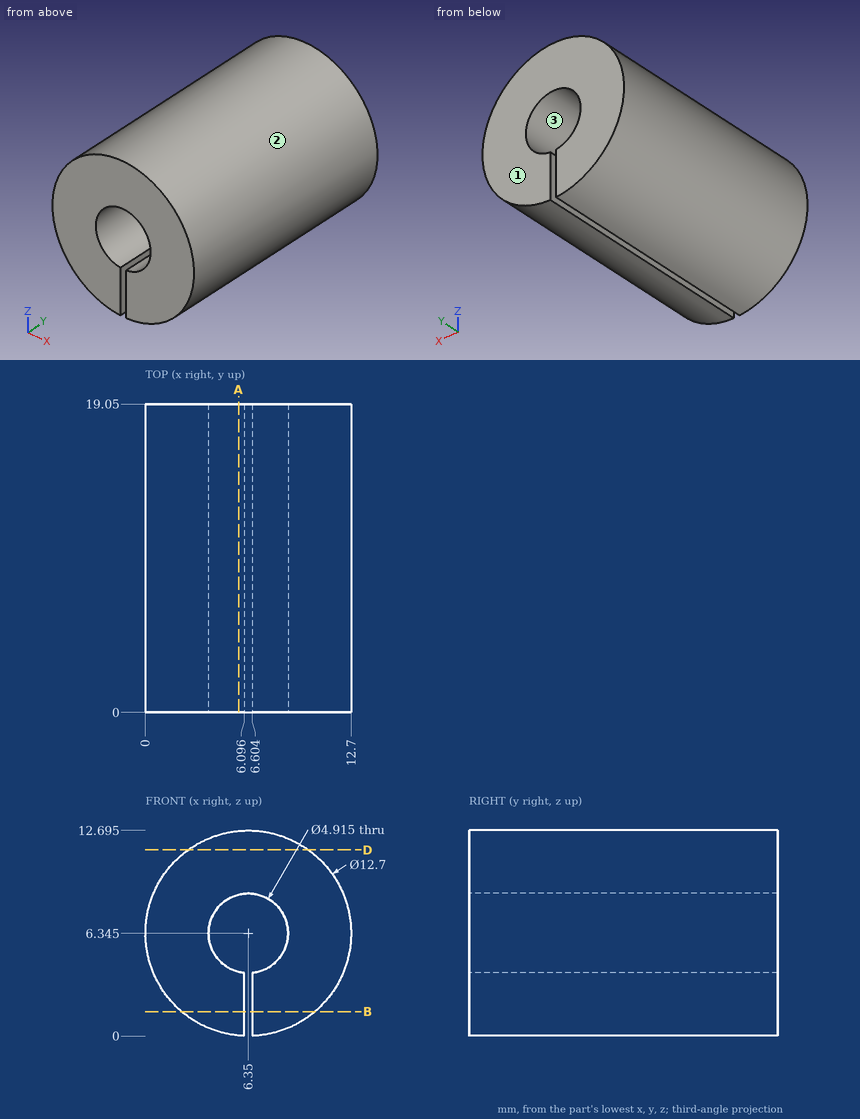
Here's the drawing with two shaded views (mm, measured from the low corner). I have some questions. Coordinates: 2 decimals unless noted, no trailing zeros. Order: outer loops, then holes, each group sorted by start corner. A loop starts at its lowest first (then second) coordinate and runs counter-clockwise, first axis right, second up. Notation, with made-up numbers: (59, 84) - (88, 84) arc R24 cw to (88, 118) - close; hole circle Ø9 at (-25.75, -4.5). An arc over 180 degrees is marked (long way). Answer in a Markdown table with one row per item. Add a question column.
(1) If we section it at B-B, the plane z = 1.5: Please give me the cut outline in (x, y).
(2) If we mould it in two halves opening along X, with no side actions, what happens to the marked faces 1, 2 and 3? For each: released by +X, released by -X, zero draft, split by the parting line, or undercut.
(3) If we section it at D-D, the plane z = 11.5: Please give me the cut outline in (x, y), then the cut area to 3 significant figures.
(4) Will these pins go through, and if not, where does the flat tip stop? pin 1 (6 mm diameter, centred on y = 8, z = 10.5, fed in from -X); pin 2 (4 mm diameter, centred on x = 6.35, z = 6.34, fed in from +Y); pin 3 (6 mm diameter, centred on y = 14.5, z = 2.5, fed in from +X); pin 4 (1 mm diameter, centred on y = 4, z = 2.5, fed in from +X).
(5) If we section it at A-A, the plane x = 5.75: Please give me the cut outline in (y, z).
(6) I need wall thicknesses on L1, parallel to X at y = 8, z = 6.5; L2, parallel to Z at x = 6.35, y = 4 (1 decimal); L3, parallel to X at y = 15.25, z = 1. Which ranges of each line are inside material? Lowest first, please.
Results are:
| question | item | result |
|---|---|---|
| 1 | outline | (2.25, 0) - (6.1, 0) - (6.1, 19.05) - (2.25, 19.05) - close; (6.6, 0) - (10.45, 0) - (10.45, 19.05) - (6.6, 19.05) - close |
| 2 | face 1 | zero draft |
| 2 | face 2 | split by the parting line |
| 2 | face 3 | undercut |
| 3 | outline | (2.64, 0) - (10.06, 0) - (10.06, 19.05) - (2.64, 19.05) - close |
| 3 | area | 141 mm2 |
| 4 | pin 1 | stops at x = 0.11 |
| 4 | pin 2 | passes through |
| 4 | pin 3 | stops at x = 12.64 |
| 4 | pin 4 | stops at x = 11.75 |
| 5 | outline | (0, 0.02) - (19.05, 0.02) - (19.05, 3.96) - (0, 3.96) - close; (0, 8.73) - (19.05, 8.73) - (19.05, 12.67) - (0, 12.67) - close |
| 6 | L1 | x = 0 to 3.9, 8.8 to 12.7 |
| 6 | L2 | z = 8.8 to 12.7 |
| 6 | L3 | x = 2.92 to 6.1, 6.6 to 9.78 |
